Autodesk Inventor part; units mm, degrees
ref_plane "YZ Plane" through (0, 0, 0) normal (1, 0, 0) x (0, 1, 0)
ref_plane "XZ Plane" through (0, 0, 0) normal (0, 1, 0) x (-1, 0, 0)
ref_plane "XY Plane" through (0, 0, 0) normal (0, 0, 1) x (1, 0, 0)
sketch "Sketch1" plane through (0, 0, 0) normal (0, 0, 1) x (1, 0, 0)
  line L0 (-21.15, -21.15) -> (21.15, -21.15)
  line L1 (21.15, -21.15) -> (21.15, 21.15)
  line L2 (21.15, 21.15) -> (-21.15, 21.15)
  line L3 (-21.15, 21.15) -> (-21.15, -21.15)
  line L4 (-21.15, -21.15) -> (21.15, 21.15) construction
  line L5 (21.15, -21.15) -> (-21.15, 21.15) construction
  circle A0 centre (0, 0) radius 18
  dimension "d0" = 42.3
  dimension "d1" = 42.3
  dimension "d2" = 36
extrude "Extrusion1" add sketch "Sketch1" against normal blind 40 contours L3 L2 L1 L0 | A0
extrude "Extrusion2" add sketch "Sketch1" along normal blind 27.3 contours A0
sketch "Sketch2" plane through (0, 0, 27.3) normal (0, 0, 1) x (1, 0, 0)
  circle A0 centre (0, 0) radius 4
  dimension "d7" = 8
extrude "Extrusion3" add sketch "Sketch2" along normal blind 20
properties part number "gearedNema17"
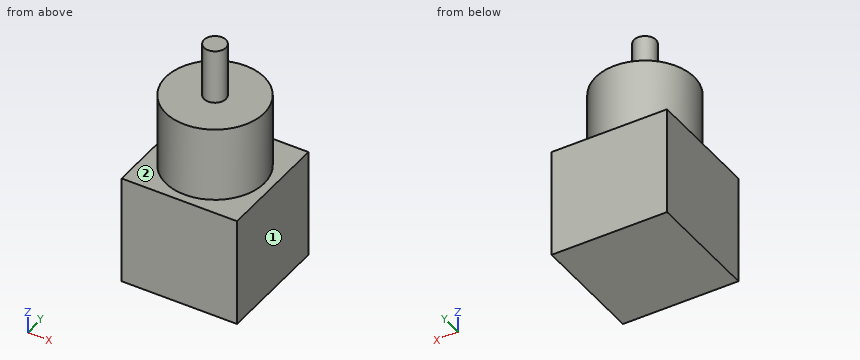
Geometry: final body of the model. Coordinates: model frame, mm. Face numbers are marked on the shaded views. A direction names the side the tool comes from. Round coordinates to 2 decimals unless told otherwise and drop trailing zeros. Order: outer loops, then holes, each group sorted by start corner. A loop starts at its lowest first (then second) coordinate and runs counter-clockwise, first axis right, second up. Notation, with made-up numbers: (22, 60) -> (59, 60) arc R27 ccw to (59, 96) -> close; hole circle Ø11 at (8, 10.25). An arc over 180 degrees is marked (long way). Put each result on its own line as item: value. Start each with the question number.
Q1. Section A-A on y = 0. Return the cut outline in (x, z), and give its area (3 significant figures).
Q2. Reachability of the marked faces 1 and 2 from +Z, -Z, +X, -X, +Y, -Y: full face, straight path, thin tool, end or side. Return the list, or none.
Q3. First-contact query: pin 1 (3 mm diameter, centred on y = 6.5, z = 14.5, fed in from -X); pin 2 (6 mm diameter, centred on x = 2, z = 24, fed in from +Y). Flat tips, straight axial feed; report the tip coordinate or a pass-through.
Q4. Section D-D on x = 16.5. Return the cut outline in (y, z).
Q5. Line query: probe 1 along Z at (x, y) = (-4.5, 3); probe 2 along Y at (x, z) = (0, 37); probe 3 along Z at (x, y) = (-15, 12). Output: solid intervals per line, ascending.
Q6. Section C-C on z = 25.5. Return the cut outline in (x, y), and give its area (3 significant figures).
Ans:
1. outline: (-21.15, -40) -> (21.15, -40) -> (21.15, 0) -> (18, 0) -> (18, 27.3) -> (4, 27.3) -> (4, 47.3) -> (-4, 47.3) -> (-4, 27.3) -> (-18, 27.3) -> (-18, 0) -> (-21.15, 0) -> close
1. area: 2,830 mm2
2. face 1: +Z, -Z, +X, +Y, -Y
2. face 2: +Z
3. pin 1: stops at x = -17.29
3. pin 2: stops at y = 18
4. outline: (-21.15, -40) -> (21.15, -40) -> (21.15, 0) -> (7.19, 0) -> (7.19, 27.3) -> (-7.19, 27.3) -> (-7.19, 0) -> (-21.15, 0) -> close
5. probe 1: z = -40 to 27.3
5. probe 2: y = -4 to 4
5. probe 3: z = -40 to 0
6. outline: circle Ø36 at (0, 0)
6. area: 1,020 mm2
